```python
from build123d import *

# Parameters (mm, degrees)
SKETCH1_W               = 32.639
SKETCH1_H               = 71.755
BOSS_EXTRUDE1_DEPTH     = 4.064
SKETCH2_W               = 26.924
SKETCH2_H               = 19.304
SKETCH2_W_2             = 22.479
SKETCH2_H_2             = 9.144
BOSS_EXTRUDE2_DEPTH     = 10.795
SKETCH3_W               = 17.78
SKETCH3_H               = 21.336
BOSS_EXTRUDE3_DEPTH     = 9.906
CUT_EXTRUDE1_DEPTH      = 66.282848799
CUT_EXTRUDE1_DEPTH_BACK = 66.282848799
SKETCH4_W               = 13.716
SKETCH4_H               = 8.001
SKETCH4_W_2             = 12.5984


with BuildPart() as part:
    # Sketch1 → Boss-Extrude1 (new body)
    with BuildSketch(Plane(origin=(0, 0, 0), x_dir=(1, 0, 0), z_dir=(0, 1, 0))):
        Rectangle(SKETCH1_W, SKETCH1_H)
    extrude(amount=BOSS_EXTRUDE1_DEPTH)

    # Sketch2 → Boss-Extrude2 (add)
    with BuildSketch(Plane(origin=(0, 4.064, 0), x_dir=(1, 0, 0), z_dir=(0, 1, 0))):
        with Locations((2.0955, 21.9075)):
            Rectangle(SKETCH2_W, SKETCH2_H)
        Polygon((15.5575, 12.2555), (-11.3665, 12.2555), (-17.7165, 12.2555), (-17.7165, -5.9309), (-14.7955, -5.9309), (-6.9215, -5.9309), (18.0975, -5.9309), (18.0975, 12.2555), align=None)
        Polygon((-6.9215, -5.9309), (-14.7955, -5.9309), (-14.7955, -29.5275), (-6.9215, -29.5275), (-6.9215, -20.3835), align=None)
        with Locations((4.318, -24.9555)):
            Rectangle(SKETCH2_W_2, SKETCH2_H_2)
    extrude(amount=BOSS_EXTRUDE2_DEPTH)

    # Sketch3 → Boss-Extrude3 (add)
    with BuildSketch(Plane(origin=(0, 4.064, 0), x_dir=(1, 0, 0), z_dir=(0, 1, 0))):
        with Locations((0, -43.4975)):
            Rectangle(SKETCH3_W, SKETCH3_H)
    extrude(amount=BOSS_EXTRUDE3_DEPTH)

    # Sketch4 → Cut-Extrude1 (cut, two sides: drawn at the far end of the back side and taken through both)
    with BuildSketch(Plane(origin=(15.5575, 0, 0), x_dir=(0, 0, -1), z_dir=(1, 0, 0)).offset(-CUT_EXTRUDE1_DEPTH_BACK)):
        with Locations((21.9075, 8.0645)):
            Rectangle(SKETCH4_W, SKETCH4_H)
        with Locations((3.1623, 8.0645)):
            Rectangle(SKETCH4_W_2, SKETCH4_H)
    extrude(amount=CUT_EXTRUDE1_DEPTH + CUT_EXTRUDE1_DEPTH_BACK, mode=Mode.SUBTRACT)


solid = part.part
```
For this review, take the finished solid that the model builds, in its own axes (mm). A direction names the side the tool comes from. Coordinates: 2 decimals unless noted, no trailing zeros. Write each loop counter-clockwise with the first axis right and the second up, starting at its lowest first coordinate (ties: lowest second). Pieces come first, ordered by that corner, then holes.
(1) For pin 1 Ø5.5 at (x, z) = (-1, 46) entering from -Y; pin 2 Ø14 at (x, z) = (3.5, 40) entering from +Y; pin 3 Ø8 at (y, z) = (8.5, 32) entering from +X, all flat-tipped, find the tip position at first contact; note any pin that passes through.
(2) Add section C-C on z = -4. Give the boundary of the cut face in (x, y) (1 decimal).
(3) Tool access review of faces 4 (the face through (17, 4.064, -11)), 5 (the face through (2, 12.065, -22)), 6 (the face through (-11.366, 13, -22)), 7 (the face through (0, 9, 32.83)): name each direction out of +Z, -Z, +X, -X, +Y, -Y from which nothing blocks a thin tool from reaching the whole face with its end or side.
(4) Add section A-A on y = 6.75. Give the boundary of the cut face in (x, z).
(5) Add section D-D on y = 13. Give the boundary of the cut face in (x, z), then the cut area to 3 significant figures.
(6) The part is to be moulded in two halves that separate along Z. For faces 1 (the face through (0, 8, -9.462)), 2 (the face through (16.32, 2, 1)), 3 (the face through (0, 2, -35.878)), say which applies: +Z half, -Z half, draft (parallel to the pull), parting line (faces both ways), or undercut.
(7) Wall thickness on probe 1 along Z at (x, y) = (-6, 11.25); probe 2 along Z at (x, y) = (-2, 13.25); probe 3 along Z at (x, y) = (12, 9.5): over which ranges is each line inside the solid? List them lowest first.
(8) Add section B-B on x = 10.5. Give the boundary of the cut face in (y, z) (1 decimal).
Answer sheet:
1. pin 1: stops at y = 4.06
1. pin 2: stops at y = 13.97
1. pin 3: stops at x = 15.56
2. outline: (-17.7, 12.1) - (18.1, 12.1) - (18.1, 14.9) - (-17.7, 14.9) - close; (-16.3, 0) - (16.3, 0) - (16.3, 4.1) - (-16.3, 4.1) - close
3. face 4: +Z, -Z, +X, -Y
3. face 5: +X, -X
3. face 6: -Z, -X, +Y
3. face 7: +X, -X, +Y
4. outline: (-17.72, -12.26) - (-11.37, -12.26) - (-11.37, -15.05) - (15.56, -15.05) - (15.56, -12.26) - (18.1, -12.26) - (18.1, -9.46) - (-17.72, -9.46) - close; (-17.72, 3.14) - (18.1, 3.14) - (18.1, 5.93) - (-6.92, 5.93) - (-6.92, 20.38) - (15.56, 20.38) - (15.56, 29.53) - (-14.8, 29.53) - (-14.8, 5.93) - (-17.72, 5.93) - close; (-11.37, -31.56) - (15.56, -31.56) - (15.56, -28.77) - (-11.37, -28.77) - close; (-8.89, 32.83) - (8.89, 32.83) - (8.89, 54.17) - (-8.89, 54.17) - close
5. outline: (-17.72, -12.26) - (-11.37, -12.26) - (-11.37, -31.56) - (15.56, -31.56) - (15.56, -12.26) - (18.1, -12.26) - (18.1, 5.93) - (-6.92, 5.93) - (-6.92, 20.38) - (15.56, 20.38) - (15.56, 29.53) - (-14.8, 29.53) - (-14.8, 5.93) - (-17.72, 5.93) - close; (-8.89, 32.83) - (8.89, 32.83) - (8.89, 54.17) - (-8.89, 54.17) - close
5. area: 1,940 mm2
6. face 1: undercut
6. face 2: draft
6. face 3: -Z half
7. probe 1: z = -31.56 to -28.77, -15.05 to -9.46, 3.14 to 5.93, 20.38 to 29.53, 32.83 to 54.17
7. probe 2: z = -31.56 to 5.93, 20.38 to 29.53, 32.83 to 54.17
7. probe 3: z = -31.56 to -28.77, -15.05 to -9.46, 3.14 to 5.93, 20.38 to 29.53
8. outline: (0, -35.9) - (4.1, -35.9) - (4.1, -31.6) - (14.9, -31.6) - (14.9, 5.9) - (4.1, 5.9) - (4.1, 20.4) - (14.9, 20.4) - (14.9, 29.5) - (4.1, 29.5) - (4.1, 35.9) - (0, 35.9) - close; hole (4.1, -28.8) - (12.1, -28.8) - (12.1, -15) - (4.1, -15) - close; hole (4.1, -9.5) - (12.1, -9.5) - (12.1, 3.1) - (4.1, 3.1) - close
